Build history of the part. All positions in model axes, mm. Give positions to 0.01 mm unless a question says otherwise; leave off trailing zeros. Order: outer loops, then holes, each group sorted by start corner. A loop starts at its lowest first (then second) coordinate and runs counter-clockwise, first axis right, second up. Notation, with made-up numbers: (-29.5, -2.5) - (-14.5, -2.5) arc R16 cw to (-14.5, 6.5) - close; hole circle Ø9 at (-7, 58.5). An arc over 180 degrees is marked (long way). Write each question's results on one line, items separated by ' | '. Start each with the question number.
1) Drop flat-ended pins along their axis: pin 1 Ø1.5 at (x, z) = (51, 0.5) entering from -Y; pin 2 Ø9 at (x, y) = (80.11, 46.25) entering from +Z; pin 3 Ø1.5 at (y, z) = (-13.5, 2.5) entering from -X. Give the stop position or say it passes through.
2) Cut at C-C on z = 1.5. List the corners of the cut face in (x, y).
3) Cut at A-A on x = 0. List the corners of the cut face in (y, z).
4) Two-plate mould, pull along Y, no slides. Class faces 1 (the face through (-22.22, 100.063, 1.479)), 2 (the face through (-84.075, 43.208, 1.521)), 3 (the face through (1.08, 97.38, 1.52)), 4 (the face through (0, -83, 3)): +Y half, -Y half, draft (parallel to the pull), parting line (faces both ways), or undercut.
5) Cut at D-D on y = -46.25. List the corners of the cut face in (x, z).
6) Drill centre lines: line 1 along Y through (x, z) = (0, 2.05); line 2 along X through (y, z) = (-47.5, 0.4); line 3 along Y through (x, z) = (71.5, 2.5). Where is each one in solid material? Low to high. Write a range as from..to.
7) Cut at B-B on y = -68. List the corners of the cut face in (x, z), plus the area to 3 significant figures.
Autodesk Inventor part; units mm, degrees
ref_plane "YZ Plane" through (0, 0, 0) normal (1, 0, 0) x (0, 1, 0)
ref_plane "XZ Plane" through (0, 0, 0) normal (0, 1, 0) x (-1, 0, 0)
ref_plane "XY Plane" through (0, 0, 0) normal (0, 0, 1) x (1, 0, 0)
sketch "Sketch1" plane through (0, 0, 0) normal (0, 0, 1) x (1, 0, 0)
  circle A0 centre (0, 0) radius 82.5
  circle A1 centre (0, 0) radius 102.5
  circle A2 centre (0, 0) radius 92.5 construction
  line L0 (0, 102.5) -> (0, 82.5) construction
  point P0 (0, 92.5)
  dimension "d30" = 165
  dimension "d32" = 205
extrude "Plate1" add sketch "Sketch1" along normal blind 3
sketch "Sketch2" plane through (0, 0, 3) normal (0, 0, 1) x (1, 0, 0)
  circle A0 centre (0, 0) radius 82.5 construction
  circle A1 centre (0, 0) radius 102.5 construction
  circle A2 centre (0, 0) radius 102.5 construction
  circle A3 centre (0, 0) radius 82.5 construction
  circle A4 centre (0, -92.5) radius 5
  circle A5 centre (0, 0) radius 92.5 construction
  dimension "d31" = 185
  dimension "d21" = 10
extrude "Extrusion1" cut sketch "Sketch2" against normal through all
pattern_circular "Circular Pattern2" count 6 over 360 about axis through (0, 0, 0) along (0, 0, 1) of "Extrusion1"
equation "\"d30\" = back_steel_circle_внутр_диам"
equation "\"d32\" = back_steel_circle_внутр_диам + back_steel_circle_ширина_кольца"
equation "\"d31\" = back_steel_circle_диам_центров"
equation "\"d21\" = back_steel_circle_диам_шпильки"
equation "\"d2\" = Thickness"
equation "\"BendRadius\" = Thickness"
equation "\"BendReliefWidth\" = Thickness"
equation "\"BendReliefDepth\" = 0.5 * Thickness"
equation "\"CornerReliefSize\" = 4 * Thickness"
equation "\"MinimumRemnant\" = 2 * Thickness"
equation "\"TransitionRadius\" = BendRadius"
equation "\"JacobiRadiusSize\" = BendRadius"
equation "\"GapSize\" = Thickness"
equation "\"back_steel_circle_диам_центров\" = back_steel_circle_внутр_диам + 0.5 * back_steel_circle_ширина_кольца"
equation "\"back_steel_circle_диам_шпильки\" = 10"
equation "\"back_steel_circle_проходной_диаметр\" = 125"
properties part number "NVPH-321 joint steel ring"
Results:
1) pin 1: y = -89.34 | pin 2: through | pin 3: x = -101.7
2) outline: circle Ø205 at (0, 0); hole circle Ø10 at (-80.11, -46.25); hole circle Ø10 at (-80.11, 46.25); hole circle Ø165 at (0, 0); hole circle Ø10 at (0, -92.5); hole circle Ø10 at (0, 92.5); hole circle Ø10 at (80.11, -46.25); hole circle Ø10 at (80.11, 46.25)
3) outline: (-102.5, 0) - (-97.5, 0) - (-97.5, 3) - (-102.5, 3) - close; (-87.5, 0) - (-82.5, 0) - (-82.5, 3) - (-87.5, 3) - close; (82.5, 0) - (87.5, 0) - (87.5, 3) - (82.5, 3) - close; (97.5, 0) - (102.5, 0) - (102.5, 3) - (97.5, 3) - close
4) face 1: parting line | face 2: undercut | face 3: undercut | face 4: draft
5) outline: (-91.47, 0) - (-85.11, 0) - (-85.11, 3) - (-91.47, 3) - close; (-75.11, 0) - (-68.32, 0) - (-68.32, 3) - (-75.11, 3) - close; (68.32, 0) - (75.11, 0) - (75.11, 3) - (68.32, 3) - close; (85.11, 0) - (91.47, 0) - (91.47, 3) - (85.11, 3) - close
6) line 1: -102.5..-97.5, -87.5..-82.5, 82.5..87.5, 97.5..102.5 | line 2: -90.83..-84.95, -75.27..-67.45, 67.45..75.27, 84.95..90.83 | line 3: -73.44..-41.16, 41.16..73.44
7) outline: (-76.7, 0) - (-46.71, 0) - (-46.71, 3) - (-76.7, 3) - close; (46.71, 0) - (76.7, 0) - (76.7, 3) - (46.71, 3) - close | area: 180 mm^2
